Here's how the part is built. I have some questions about the finished solid (model axes, mm). Round coordinates to 2 decimals unless told otherwise and drop trailing zeros. Loops run counter-clockwise (first coordinate to the right, second up) from the corner with the lowest first, then second, coordinate; pieces in that order, holes last. Notation, with made-up numbers: (43.5, 58.25) - (54.5, 58.25) arc R28 cw to (54.5, 93.25) - close; hole circle Ø4 at (-9.75, 46). An arc over 180 degrees is marked (long way). Answer as a JSON object with one key per item and string values. Group by question number.
1) Will this pin go through, and if not, where does the flat tip stop? P1, Ø9, axis at x = -43.51, y = 83.13, coming from the +Z side.
2) I want a section at A-A, the plane x = -42.5. Please give me the cut outline in (y, z), then the cut area to 3 significant figures.
3) If I drill on line 1 along Y through (x, z) = (-183.5, 2.25); line 2 along X through (y, z) = (122.5, 2.1); line 3 along Y through (x, z) = (-86, 3.05), over which ranges is the centre line in solid material (lowest first)? Write a range as [from, to].
4) If we mould it in two halves opening along Y, with no side actions, what happens to faces 1 (the face through (-39.54, 51.175, 2.028)), 2 (the face through (-117, 131.278, 2)), 3 (the face through (-207.749, 81, 2))? For each: pulls with the +Y half, pulls with the -Y half, needs draft (parallel to the pull), parting line crosses it, or undercut.
5) I want a section at B-B, the plane z = 0.9. Give the number of separate pieces and of enclosed holes in the cut face, then the cut area to 3 significant figures.
Autodesk Fusion 360 part; units mm, degrees
box "BoxPrimitive1" add length 100 width 185 height 4 placed x (0, -1, 0) y (1, 0, 0) z (0, 0, 1) at (-207.7492, 131.2779, 0)
sketch "Sketch2" plane through (0, 0, 4) normal (0, 0, 1) x (-1, 0, 0)
  line L0 (207.7492, -31.2779) -> (22.7492, -31.2779)
  line L1 (22.7492, -31.2779) -> (22.7492, -131.2779)
  line L2 (22.7492, -131.2779) -> (207.7492, -131.2779)
  line L3 (207.7492, -131.2779) -> (207.7492, -31.2779)
  circle A0 centre (43.5078, -48.1327) radius 5
  circle A1 centre (90.1744, -48.1327) radius 5
  circle A2 centre (136.8411, -48.1327) radius 5
  circle A3 centre (183.5078, -48.1327) radius 5
  circle A4 centre (43.5078, -83.1327) radius 5
  circle A5 centre (43.5078, -118.1327) radius 5
  circle A6 centre (90.1744, -83.1327) radius 5
  circle A7 centre (136.8411, -83.1327) radius 5
  circle A8 centre (183.5078, -83.1327) radius 5
  circle A9 centre (90.1744, -118.1327) radius 5
  circle A10 centre (136.8411, -118.1327) radius 5
  circle A11 centre (183.5078, -118.1327) radius 5
  dimension "d7" = 10
  dimension "d10" = 140
  dimension "d11" = 0
  dimension "d14" = 0
  dimension "d15" = -70
  dimension "d18" = 140
  dimension "d19" = 0
  dimension "d22" = 140
  dimension "d23" = 0
extrude "Extrude1" cut sketch "Sketch2" against normal blind 5 contours A0 | A1 | A2 | A3 | A4 | A5 | A6 | A7 | A8 | A9 | A10 | A11
Outcome:
{
 "1": {"P1": "through"},
 "2": {"outline": "(31.28, 0) - (43.24, 0) - (43.24, 4) - (31.28, 4) - close; (53.03, 0) - (78.24, 0) - (78.24, 4) - (53.03, 4) - close; (88.03, 0) - (113.24, 0) - (113.24, 4) - (88.03, 4) - close; (123.03, 0) - (131.28, 0) - (131.28, 4) - (123.03, 4) - close", "area": "282 mm^2"},
 "3": {"line 1": "[31.28, 43.13], [53.13, 78.13], [88.13, 113.13], [123.13, 131.28]", "line 2": "[-207.75, -185.94], [-181.07, -139.28], [-134.41, -92.61], [-87.74, -45.94], [-41.07, -22.75]", "line 3": "[31.28, 45.38], [50.88, 80.38], [85.88, 115.38], [120.88, 131.28]"},
 "4": {"face 1": "undercut", "face 2": "pulls with the +Y half", "face 3": "needs draft"},
 "5": {"separate pieces": "1", "enclosed holes": "12", "area": "17,600 mm^2"}
}
